Autodesk Inventor part; units mm, degrees
ref_plane "YZ Plane" through (0, 0, 0) normal (1, 0, 0) x (0, 1, 0)
ref_plane "XZ Plane" through (0, 0, 0) normal (0, 1, 0) x (-1, 0, 0)
ref_plane "XY Plane" through (0, 0, 0) normal (0, 0, 1) x (1, 0, 0)
sketch "Эскиз1" plane through (0, 0, 0) normal (0, 0, 1) x (1, 0, 0)
  line L0 (27.5467, -7.6681) -> (1.5467, -7.6681)
  line L1 (-6.4533, -7.6681) -> (-34.4903, -7.6681)
  line L2 (-34.4903, -7.6681) -> (-6.4533, -7.6681)
  line L3 (1.5467, -7.6681) -> (27.5467, -7.6681)
  line L4 (27.5467, -7.6681) -> (27.5467, 28.4819)
  line L5 (27.5467, 28.4819) -> (-2.4533, 28.4819)
  line L6 (-2.4533, 28.4819) -> (-34.4903, 28.4819)
  line L7 (-34.4903, 28.4819) -> (-34.4903, -7.6681)
  line L8 (-34.4903, 13.2319) -> (-34.4903, 5.0319)
  line L9 (-34.4903, 3.2319) -> (-34.4903, -7.6681)
  circle A0 centre (11.5467, 9.1319) radius 1.575
  circle A1 centre (-2.4533, 24.4819) radius 1.6
  line L10 (-6.4533, -7.6681) -> (1.5467, -7.6681)
  line L11 (-16.4718, -11.6681) -> (-16.4718, -18.4681)
  line L12 (9.5282, -11.6681) -> (9.5282, -18.4681)
  line L13 (-16.4718, -18.4681) -> (9.5282, -18.4681)
  circle A2 centre (-38.4903, -7.6681) radius 1.6
  circle A3 centre (31.5467, -7.6681) radius 1.6
  arc A4 (31.5467, -11.6681) -> (27.5467, -7.6681) centre (31.5467, -7.6681) ccw
  line L14 (27.5467, -7.6681) -> (9.5282, -7.6681)
  arc A5 (-34.4903, -7.6681) -> (-38.4718, -11.6681) centre (-38.4903, -7.6681) ccw
  arc A6 (-38.4718, -11.6681) -> (-38.4533, -11.6681) centre (-38.4533, -7.6681) ccw
  line L15 (-38.4533, -11.6681) -> (-34.4903, -11.6681)
  arc A7 (-19.6718, -21.6681) -> (-34.4903, -11.6681) centre (-35.1698, -28.6545) ccw
  line L16 (12.7282, -21.6681) -> (-19.6718, -21.6681)
  arc A8 (27.5467, -11.6681) -> (12.7282, -21.6681) centre (28.2263, -28.6545) ccw
  line L17 (27.5467, -11.6681) -> (31.5467, -11.6681)
  arc A9 (35.5467, -7.6681) -> (27.5467, -7.6681) centre (31.5467, -7.6681) ccw
  line L18 (35.5467, 28.4819) -> (35.5467, -7.6681)
  line L19 (35.5467, 28.4819) -> (-2.4533, 28.4819)
  circle A10 centre (-2.4533, 24.4819) radius 4
  line L20 (-2.4533, 28.4819) -> (-42.4533, 28.4819)
  line L21 (-42.4533, -7.1253) -> (-42.4533, 28.4819)
  arc A11 (-34.4903, -7.6681) -> (-42.4533, -7.1253) centre (-38.4903, -7.6681) ccw
  line L22 (-34.4903, -7.6681) -> (27.5467, -7.6681)
  arc A12 (-34.4903, 3.2319) -> (-34.4903, 5.0319) centre (-30.4903, 4.1319) ccw
  line L23 (-34.4903, 3.2319) -> (-34.4903, 5.0319)
  line L24 (-34.4903, 13.2319) -> (-34.4903, 15.0319)
  arc A13 (-34.4903, 13.2319) -> (-34.4903, 15.0319) centre (-30.4903, 14.1319) ccw
  circle A14 centre (17.5097, 4.1319) radius 4.1
  circle A15 centre (-16.4533, 9.1319) radius 7
  circle A16 centre (11.5467, 9.1319) radius 3.5
  circle A17 centre (17.5097, 14.1319) radius 4.1
  line L25 (35.5467, 28.4819) -> (27.5467, 28.4819)
  line L26 (27.5467, 28.4819) -> (27.5467, -11.6681)
  line L27 (27.5467, -11.6681) -> (35.5467, -11.6681)
  line L28 (35.5467, -11.6681) -> (35.5467, 28.4819)
  line L29 (-42.4533, 28.4819) -> (-34.4903, 28.4819)
  line L30 (-34.4903, 28.4819) -> (-34.4903, -11.6681)
  line L31 (-34.4903, -11.6681) -> (-42.4533, -11.6681)
  line L32 (-42.4533, -11.6681) -> (-42.4533, 28.4819)
  line L33 (27.5467, -11.6681) -> (-34.4903, -11.6681)
  line L34 (-34.4903, -11.6681) -> (-34.4903, -7.6681)
  line L35 (-34.4903, -7.6681) -> (27.5467, -7.6681)
  line L36 (27.5467, -7.6681) -> (27.5467, -11.6681)
  line L37 (9.5282, -7.6681) -> (9.5282, -11.6681)
  line L38 (-16.4718, -11.6681) -> (-16.4718, -7.6681)
  line L39 (-16.4718, -7.6681) -> (-34.4903, -7.6681)
  point P0 (0, 0)
  point P1 (-2.4533, -2.0181)
  point P2 (1.5467, -7.6681)
  point P3 (-42.4533, -8.2109)
extrude "Выдавливание1" add sketch "Эскиз1" along normal blind 3.2 contours L26 L33 L37 L0 | A10 | L0 L10 L1 L7 A12 A13 L6 L5 L4 | L4 L19 L18 A4 | A4 L17 L26 | L37 L33 L38 L1 L10 L0 | L33 L30 L1 L38 | L7 A5 L21 L20 | L15 A6 A5 L32 L30 | A13 L7 | L32 A5 | L7 A12 | A14 | A15 | A16 | A17
sketch "Эскиз2" plane through (0, 0, 3.2) normal (0, 0, 1) x (1, 0, 0)
  line L0 (-16.4718, -7.6681) -> (-13.4718, -7.6681)
  line L1 (6.5282, -7.6681) -> (9.5282, -7.6681)
  line L2 (-38.4533, -11.6681) -> (31.5467, -11.6681)
  line L3 (9.5282, -11.6681) -> (-16.4718, -11.6681)
  line L4 (-16.4718, -11.6681) -> (-16.4718, -7.6681)
  line L5 (-16.4718, -7.6681) -> (9.5282, -7.6681)
  line L6 (9.5282, -7.6681) -> (9.5282, -11.6681)
  line L7 (-16.4718, -7.6681) -> (9.5282, -7.6681)
  line L8 (9.5282, -7.6681) -> (9.5282, 2.3319)
  line L9 (9.5282, 2.3319) -> (-16.4718, 2.3319)
  line L10 (-16.4718, 2.3319) -> (-16.4718, -7.6681)
  point P0 (0, 0)
  point P1 (-16.4718, -11.6681)
  dimension "d4" = 26
  dimension "d5" = 10
extrude "Выдавливание2" cut sketch "Эскиз2" against normal blind 3.2
fillet "Сопряжение1" radius 2 2 edges at (9.5282, 2.3319, 1.6) (-16.4718, 2.3319, 1.6)
properties part number "крышка захвата"
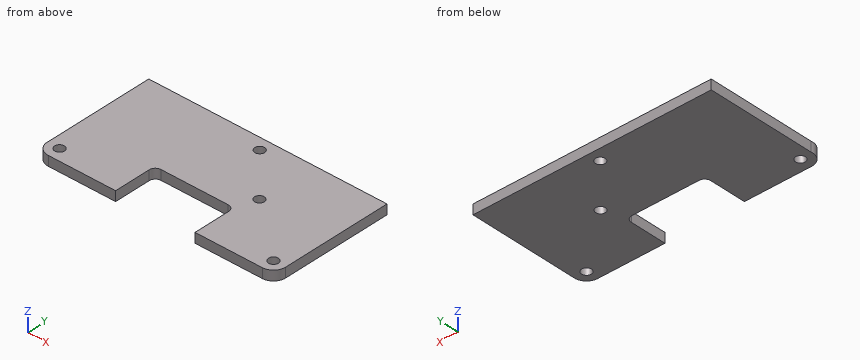
Input: part model. Units: mm. Frame: model coordinates. Give positions to 0.01 mm unless a question says otherwise; leave off trailing zeros. Order: outer loops, then holes, each group sorted by start corner. A loop starts at its lowest first (then second) coordinate and runs counter-clockwise, first axis right, second up. Notation, with made-up numbers: M 5,5 L 21,5 A27 cw 21,25 Z; hole C 89,65 d6. An arc over 180 degrees is marked long. Return JSON: item names as keys, results as strings.
1) Section query B-B on x = 11. Output: boundary loops of the cut face in (y, z).
Taken from the geometry:
{"outline": "M -11.67,0 L 7.65,0 L 7.65,3.2 L -11.67,3.2 Z; M 10.61,0 L 28.48,0 L 28.48,3.2 L 10.61,3.2 Z"}
2) Section query D-D on y = -3. Output: boundary loops of the cut face in (x, z), and give its area (3 significant figures).
Taken from the geometry:
{"outline": "M -42.45,0 L -16.47,0 L -16.47,3.2 L -42.45,3.2 Z; M 9.53,0 L 35.55,0 L 35.55,3.2 L 9.53,3.2 Z", "area": "166 mm2"}
3) Contact query for flat-ended pins moving along their axis: pin 1 (3 mm diameter, centred on x = 11.55, y = 9.13, fed in from +Z); pin 2 (1 mm diameter, centred on x = -9.5, z = 2, fed in from -Y). Output: stop coordinate, or through.
Taken from the geometry:
{"pin 1": "passes through", "pin 2": "stops at y = 2.33"}
4) Line query: L1, parallel to X at y = -8.5, z = 0.5; L2, parallel to X at y = -7, z = 0.45; L3, parallel to X at y = -6, z = 0.45. Output: solid intervals per line, ascending. Write a range as [from, to].
Taken from the geometry:
{"L1": "x = [-42.4, -39.86], [-37.12, -16.47], [9.53, 30.18], [32.91, 35.46]", "L2": "x = [-42.45, -39.94], [-37.04, -16.47], [9.53, 30.09], [33, 35.55]", "L3": "x = [-42.45, -16.47], [9.53, 35.55]"}
5) Section query A-A on y = -8.5. Output: boundary loops of the cut face in (x, z).
Taken from the geometry:
{"outline": "M -42.4,0 L -39.86,0 L -39.86,3.2 L -42.4,3.2 Z; M -37.12,0 L -16.47,0 L -16.47,3.2 L -37.12,3.2 Z; M 9.53,0 L 30.18,0 L 30.18,3.2 L 9.53,3.2 Z; M 32.91,0 L 35.46,0 L 35.46,3.2 L 32.91,3.2 Z"}
6) Section query C-C on z = 1.1. Output: boundary loops of the cut face in (x, y) (3 decimals), and give its area (3 significant figures).
Taken from the geometry:
{"outline": "M -42.453,-7.125 A4 ccw -38.472,-11.668 A1.333 ccw -38.453,-11.668 L -16.472,-11.668 L -16.472,0.332 A2 cw -14.472,2.332 L 7.528,2.332 A2 cw 9.528,0.332 L 9.528,-11.668 L 31.547,-11.668 A4 ccw 35.547,-7.668 L 35.547,28.482 L -42.453,28.482 Z; hole C -38.49,-7.668 d3.2; hole C -2.453,24.482 d3.2; hole C 11.547,9.132 d3.15; hole C 31.547,-7.668 d3.2", "area": "2,730 mm2"}
